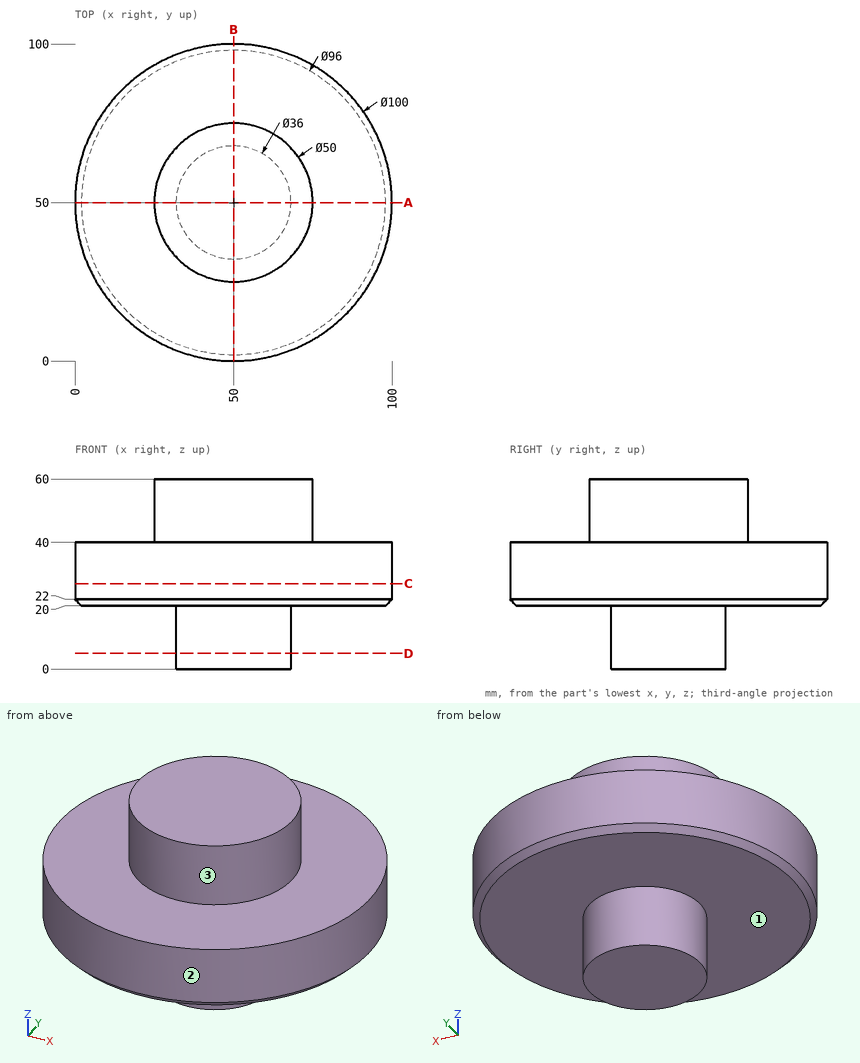
For this review, use the dimensioned drawing (mm, ordinates from the lowest corner) and the shaded views. A direction names the side the tool comes from. Coordinates: 2 decimals unless noted, no trailing zeros. Loops run counter-clockwise (first coordinate to the right, second up) from the corner with the lowest first, then second, coordinate; pieces in that order, holes last.
1. For line 1 (Y direction, x = 49, z = 36); line 2 (Z direction, x = 27, y = 74); line 3 (X direction, y = 21, z = 32.5), list the stretches that pass through material, from the lowest coordinate up.
2. Insertion check: P1, Ø12, axis at y = 14.5, z = 22.5, coming from the -X side; P2, Ø12, axis at y = 22, z = 28, coming from the -X side; P3, Ø2, axis at x = 31, z = 25, coming from the -Y side. Each pin has a flat end and moves straight along its axis. Give the tip position at first contact, or say it passes through.
3. For the marked faces 1, 2 and 3, list the 3-axis set-ups (+Z, -Z, +X, -X, +Y, -Y) from which the entire face can be reached by the end or side of a thin tool; tool diameter is ignored.
4. Add section A-A, the plane y = 50. Give the boundary of the cut face in (x, z), then the cut area to 3 significant figures.
5. Add section D-D, the plane z = 5. Give the boundary of the cut face in (x, y), then the cut area to 3 significant figures.
6. Add section C-C, the plane z = 27. Give the boundary of the cut face in (x, y).
Result:
1. line 1: y = 0.01 to 99.99
1. line 2: z = 20 to 40
1. line 3: x = 9.27 to 90.73
2. P1: stops at x = 9.63
2. P2: stops at x = 5.1
2. P3: stops at y = 3.35
3. face 1: -Z
3. face 2: +Z, -Z
3. face 3: +Z
4. outline: (0, 22) - (2, 20) - (32, 20) - (32, 0) - (68, 0) - (68, 20) - (98, 20) - (100, 22) - (100, 40) - (75, 40) - (75, 60) - (25, 60) - (25, 40) - (0, 40) - close
4. area: 3,720 mm2
5. outline: circle Ø36 at (50, 50)
5. area: 1,020 mm2
6. outline: circle Ø100 at (50, 50)
